CAD build for the part. Positions are in the model's coordinates, mm. A direction names the side the tool comes from. Round coordinates to 2 decimals unless told otherwise and drop trailing zeros. Write each loop counter-clockwise with the first axis right and the second up, starting at its lowest first coordinate (ties: lowest second). Pieces come first, ordered by that corner, then holes. Notation, with made-up numbers: (70, 75) - (118, 75) arc R29 ccw to (118, 109) - close; hole circle Ø8 at (79.25, 31.25). An arc over 180 degrees is marked (long way). Answer in a Markdown table with one row per item.
```python
from build123d import *

# Parameters (mm, degrees)
SKETCH_1_W          = 30.50790567
SKETCH_1_H          = 76
SKETCH_1_R          = 1.716069694
SKETCH_1_W_2        = 11.5
SKETCH_1_H_2        = 11.5
SKETCH_1_W_3        = 24.50790567
SKETCH_1_H_3        = 19
EXTRUDE_1_DEPTH     = 3.3
SKETCH_2_W          = 30.50790567
SKETCH_2_H          = 6
EXTRUDE_2_DEPTH     = 1
EXTRUDE_3_DEPTH     = 3.3
CUT_EXTRUDE_1_DEPTH = 3.3
EXTRUDE_5_DEPTH     = 3.3
SKETCH_6_W          = 30.50790567
SKETCH_6_H          = 24.027073242
EXTRUDE_6_DEPTH     = 3.3
CUT_EXTRUDE_3_DEPTH = 3.3
SKETCH_8_W          = 4.466233575
SKETCH_8_H          = 58.072220184
SKETCH_8_W_2        = 2.541672095
SKETCH_8_H_2        = 76
CUT_EXTRUDE_4_DEPTH = 11.3


with BuildPart() as part:
    # 草圖1 → 填料-伸長1 (new body)
    with BuildSketch(Plane.XY):
        with Locations((0, -4.833822083)):
            Rectangle(SKETCH_1_W, SKETCH_1_H)
        with Locations((-8.65, 10.166177917)):
            Circle(SKETCH_1_R, mode=Mode.SUBTRACT)
        with Locations((-0.03771926, 22.181861337)):
            Rectangle(SKETCH_1_W_2, SKETCH_1_H_2, mode=Mode.SUBTRACT)
        with Locations((8.65, 10.166177917)):
            Circle(SKETCH_1_R, mode=Mode.SUBTRACT)
        with Locations((0, -30.333822083)):
            Rectangle(SKETCH_1_W_3, SKETCH_1_H_3, mode=Mode.SUBTRACT)
    extrude(amount=EXTRUDE_1_DEPTH)

    # 草圖2 → 填料-伸長2 (add)
    with BuildSketch(Plane.XY.offset(3.3)):
        with Locations((0, 1.166177917)):
            Rectangle(SKETCH_2_W, SKETCH_2_H)
        with Locations((0, -10.833822083)):
            Rectangle(SKETCH_2_W, SKETCH_2_H)
    extrude(amount=EXTRUDE_2_DEPTH)

    # 草圖3 → 填料-伸長3 (add)
    with BuildSketch(Plane.XY):
        Polygon((15.253952835, -42.833822083), (-15.253952835, -18.474060109), (15.253952835, -18.474060109), align=None)
    extrude(amount=EXTRUDE_3_DEPTH)

    # 草圖4 → 除料-伸長1 (cut)
    with BuildSketch(Plane.XY.offset(3.3)):
        Polygon((15.253952835, -42.833822083), (-15.253952835, -18.806748841), (-15.253952835, -42.833822083), align=None)
    extrude(amount=-CUT_EXTRUDE_1_DEPTH, mode=Mode.SUBTRACT)

    # 草圖5 → 填料-伸長5 (add)
    with BuildSketch(Plane.XY.offset(3.3)):
        Polygon((15.253952835, -42.833822083), (-15.253952835, -42.833822083), (-15.253952835, -18.806748841), align=None)
    extrude(amount=-EXTRUDE_5_DEPTH)

    # 草圖6 → 填料-伸長6 (add)
    with BuildSketch(Plane.XY.offset(3.3)):
        with Locations((0, -30.820285462)):
            Rectangle(SKETCH_6_W, SKETCH_6_H)
    extrude(amount=-EXTRUDE_6_DEPTH)

    # 草圖7 → 除料-伸長3 (cut)
    with BuildSketch(Plane.XY.offset(3.3)):
        Polygon((-15.253952835, -18.833822083), (15.253952835, -42.833822083), (-15.253952835, -42.833822083), align=None)
    extrude(amount=-CUT_EXTRUDE_3_DEPTH, mode=Mode.SUBTRACT)

    # 草圖8 → 除料-伸長4 (cut)
    with BuildSketch(Plane.XY.offset(4.3)):
        with Locations((-13.020836048, 4.130067825)):
            Rectangle(SKETCH_8_W, SKETCH_8_H)
        with Locations((13.983116788, -4.833822083)):
            Rectangle(SKETCH_8_W_2, SKETCH_8_H_2)
    extrude(amount=-CUT_EXTRUDE_4_DEPTH, mode=Mode.SUBTRACT)


solid = part.part
```
Q1. Saw through at D-D on y = -32.5. List the corners of the cut face in (x, z), then the cut area to 3 significant figures.
Computed:
| item | result |
|---|---|
| outline | (2.12, 0) - (12.71, 0) - (12.71, 3.3) - (2.12, 3.3) - close |
| area | 35.0 mm2 |
Q2. 3-axis set-ups, long thin cutter, end or side, ignore diameter. For faces 4 (the flat face through (1, 16, 3.3)), 5 (the flat face through (1, -5, 3.3)), 6 (the flat face through (-5.788, 22, 2)): which of +Z, -Z, +X, -X, +Y, -Y reach the whole face in a straight line?
Computed:
| item | result |
|---|---|
| face 4 | +Z, +X, -X, +Y |
| face 5 | +Z, +X, -X |
| face 6 | +Z, -Z |
Q3. Drill centre lines: line 1 (X direction, y = 23, z = 2.05); line 2 (Z direction, x = -5.25, y = -17.5); line 3 (Y direction, x = -1.5, z = 4.05). Where is each one in solid material? Low to high.
Computed:
| item | result |
|---|---|
| line 1 | x = -10.79 to -5.79, 5.71 to 12.71 |
| line 2 | z = 0 to 3.3 |
| line 3 | y = -13.83 to -7.83, -1.83 to 4.17 |
Q4. Saw through at C-C on x = 8.65. List the corners of the cut face in (y, z).
Computed:
| item | result |
|---|---|
| outline | (-37.64, 0) - (8.45, 0) - (8.45, 3.3) - (4.17, 3.3) - (4.17, 4.3) - (-1.83, 4.3) - (-1.83, 3.3) - (-7.83, 3.3) - (-7.83, 4.3) - (-13.83, 4.3) - (-13.83, 3.3) - (-37.64, 3.3) - close; (11.88, 0) - (33.17, 0) - (33.17, 3.3) - (11.88, 3.3) - close |
Q5. Saw through at A-A on x = 3.5. List the corners of the cut face in (y, z), then the cut area to 3 significant figures.
Computed:
| item | result |
|---|---|
| outline | (-33.59, 0) - (16.43, 0) - (16.43, 3.3) - (4.17, 3.3) - (4.17, 4.3) - (-1.83, 4.3) - (-1.83, 3.3) - (-7.83, 3.3) - (-7.83, 4.3) - (-13.83, 4.3) - (-13.83, 3.3) - (-33.59, 3.3) - close; (27.93, 0) - (33.17, 0) - (33.17, 3.3) - (27.93, 3.3) - close |
| area | 194 mm2 |
Q6. Saw through at B-B on z = 1.1. List the corners of the cut face in (x, y).
Computed:
| item | result |
|---|---|
| outline | (-10.79, -22.35) - (12.71, -40.83) - (12.71, 33.17) - (-10.79, 33.17) - close; hole circle Ø3.43 at (-8.65, 10.17); hole (-5.79, 16.43) - (5.71, 16.43) - (5.71, 27.93) - (-5.79, 27.93) - close; hole circle Ø3.43 at (8.65, 10.17) |
Q7. Flat gauge pins, fed straight in: pin 1 (7 mm diameter, centred on x = 1, y = -30.5, fed in from +Z); pin 2 (0.8 mm diameter, centred on x = 6.5, z = 4, fed in from +Y); pin 3 (1.5 mm diameter, centred on x = -6, z = 3, fed in from -Y). Where does each tip first touch, or does it go through?
Computed:
| item | result |
|---|---|
| pin 1 | stops at z = 3.3 |
| pin 2 | stops at y = 4.17 |
| pin 3 | stops at y = -26.7 |
Q8. Pull direction X, two halves, no side cores. Call faces 1 (the flat face through (5.712, 22, 2)), 2 (the flat face through (1, 33.166, 2)), 3 (the flat face through (12.712, -4, 2)): released by +X, released by -X, zero draft, split by the parting line, or undercut.
Computed:
| item | result |
|---|---|
| face 1 | undercut |
| face 2 | zero draft |
| face 3 | released by +X |
